Verification items for the finished model (mm, model axes). A direction names the side the tool comes from. Round coordinates to 2 decimals unless told otherwise and drop trailing zeros. Order: outer loops, then holes, each group sorted by start corner. A loop starts at its lowest first (then second) coordinate and runs counter-clockwise, first axis right, second up. Notation, with made-up numbers: (79, 33.5) -> (102, 33.5) arc R21 cw to (102, 48.5) -> close; hole circle Ø9 at (-22.5, 67). An arc over 180 degrees is marked (long way). Put each result on its own line as item: value.
```python
from build123d import *

# Parameters (mm, degrees)
SKETCH_3_R          = 20
EXTRUDE_2_DEPTH     = 50
SKETCH_4_R          = 20
EXTRUDE_3_DEPTH     = 50
CUT_EXTRUDE_1_DEPTH = 40
CUT_EXTRUDE_2_DEPTH = 40


with BuildPart() as part:
    # Sketch 3 → Extrude 2 (new body)
    with BuildSketch(Plane(origin=(0, 0, 0), x_dir=(1, 0, 0), z_dir=(0, 1, 0))):
        with Locations(Location((0, -20, 0), (0, 0, 270))):
            Circle(SKETCH_3_R)
    extrude(amount=EXTRUDE_2_DEPTH)

    # Sketch 4 → Extrude 3 (add)
    with BuildSketch(Plane.XY):
        with Locations((0, 20)):
            Circle(SKETCH_4_R)
    extrude(amount=EXTRUDE_3_DEPTH)

    # Sketch 5 → Cut-Extrude 1 (cut)
    with BuildSketch(Plane(origin=(0, 0, 0), x_dir=(0, 0, -1), z_dir=(1, 0, 0))):
        Polygon((0, 40), (-40, 0), (-40, -16.797302677), (11.409985675, -16.797302677), align=None)
    extrude(amount=-CUT_EXTRUDE_1_DEPTH, mode=Mode.SUBTRACT)

    # Sketch 6 → Cut-Extrude 2 (cut)
    with BuildSketch(Plane.ZY):
        Polygon((0, 40), (40, 0), (42.840082068, -18.175854473), (-20.897665684, -9.087927237), align=None)
    extrude(amount=-CUT_EXTRUDE_2_DEPTH, mode=Mode.SUBTRACT)


solid = part.part
```
Item 1: Sectioned sample at D-D, the plane z = 22. Record the boundary of the cut face in (x, y), then the cut area to 3 significant figures.
Geometry check:
outline: (-19.9, 18) -> (19.9, 18) arc R20 ccw to (19.9, 22) -> (19.9, 50) -> (-19.9, 50) -> (-19.9, 22) arc R20 ccw to start
area: 1,270 mm2
Item 2: Material ranges on line 1 along X through (y, z) = (29, 47.5); line 2 along Y through (x, z) = (-9, 11); line 3 along X through (y, z) = (46, 15), recorded low to high.
Geometry check:
line 1: -17.86 to 17.86
line 2: 29 to 50
line 3: -19.36 to 19.36
Item 3: Sectioned sample at A-A, the plane x = 0. Record the boundary of the cut face in (y, z), then the cut area to 3 significant figures.
Geometry check:
outline: (0, 40) -> (40, 0) -> (50, 0) -> (50, 40) -> (40, 40) -> (40, 50) -> (0, 50) -> close
area: 1,600 mm2
Item 4: Sectioned sample at C-C, the plane x = -16. Record the boundary of the cut face in (y, z), then the cut area to 3 significant figures.
Geometry check:
outline: (8, 32) -> (32, 8) -> (50, 8) -> (50, 32) -> (32, 32) -> (32, 50) -> (8, 50) -> close
area: 1,150 mm2
Item 5: Tool access check on faces 1 (the face through (-19.98, 20.88, 41.46)), 2 (the face through (13.52, 41.46, 5.26)), 3 (the face through (0, 20, 50)). Record the directions out of +Z, -Z, +X, -X, +Y, -Y that give a thin tool (end or side, any length) a straight path to the whole face; none if there is none.
Geometry check:
face 1: +Z
face 2: +Y
face 3: +Z, +X, -X, +Y, -Y
Item 6: Sectioned sample at B-B, the plane z = 37. Record the boundary of the cut face in (x, y), then the cut area to 3 significant figures.
Geometry check:
outline: (-10.54, 3) -> (10.54, 3) arc R20 ccw to (10.54, 37) -> (10.54, 50) -> (-10.54, 50) -> (-10.54, 37) arc R20 ccw to start
area: 1,440 mm2
Item 7: Depth check by flat-ended pin: pin 1 Ø1.5 at (y, z) = (40.5, 21) entering from -X; pin 2 Ø1 at (x, z) = (-12.5, 25.5) entering from -Y; pin 3 Ø5 at (x, z) = (-14, 6) entering from -Y. Enter the tip coordinate at first touch or a pass-through.
Geometry check:
pin 1: x = -20
pin 2: y = 14
pin 3: y = 31.5
